Input: part model. Units: mm. Frame: model coordinates. Face numbers are marked on the shaded views. A direction names the side the tool comes from. Give positions to 0.01 mm unless a question says otherwise; leave off trailing zeros. Order: outer loops, then holes, each group sorted by start corner. A loop starts at its lowest first (then second) coordinate and runs counter-clockwise, first axis right, second up. Notation, with made-up numbers: (-21.5, -36) - (10.5, -36) arc R19 cw to (10.5, -23) - close; hole circle Ø6 at (-34, 2). An arc over 180 degrees is marked (long way). Answer in a Markdown table with one row per item. Add a question column.
1. Mould query, pull axis X, two halves, no side actions, for the marked faces 1 and 2. Classes: released by +X, released by -X, zero draft, split by the parting line, or undercut.
2. Access query for the marked faces 3, 4 and 5. Directions: +Z, -Z, +X, -X, +Y, -Y. A direction counts if a zero-diameter tool reaches every point of the face in a straight line with its end or side. Return the directions, or none.
3. Ray query, line 1 (X direction, y = 2.5, z = 0); line 2 (Y direction, x = -11.5, z = -3.5); line 3 (X direction, y = -2.5, z = 0). Return the intervals inside material, ascending. Write a range as [from, to].
4. Section query B-B on z = 0. Return loops of the section in (x, y), and give its area (3 significant figures).
5. Section query C-C on y = -3.75. Return loops of the section in (x, z).
6. Section query A-A on x = 0. Return loops of the section in (y, z), and give its area (3 significant figures).
7. Contact query for flat-ended pins moving along their axis: pin 1 (2 mm diameter, centred on x = 3, y = 2.5, fed in from -Z); pin 2 (2 mm diameter, centred on x = -0.5, y = 3.5, fed in from -Z); pin 3 (6 mm diameter, centred on y = 8, z = 9, fed in from -X). Output: stop coordinate, or through.
8. Section query D-D on z = 10.5. Return loops of the section in (x, y).
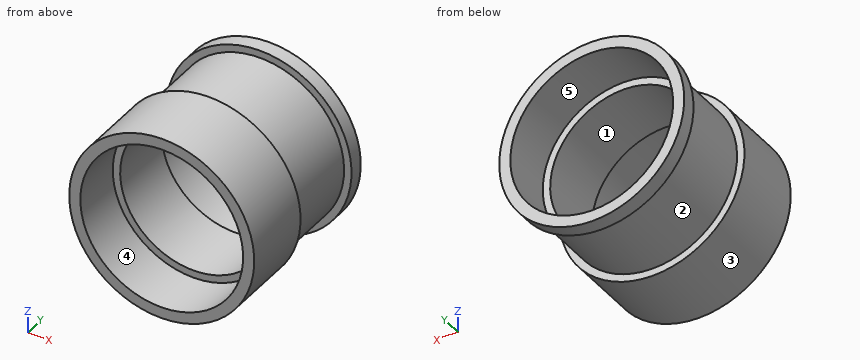
```python
from build123d import *

# Parameters (mm, degrees)
CROQUIS1_R                 = 12.5
SALIENTE_EXTRUIR1_DEPTH    = 11.5
CROQUIS2_R                 = 11
CORTAR_EXTRUIR1_DEPTH      = 7
CORTAR_EXTRUIR2_DEPTH      = 22.089096709
CORTAR_EXTRUIR2_DEPTH_BACK = 22.089096709
CROQUIS3_R                 = 10
CROQUIS4_W                 = 1
CROQUIS4_H                 = 11


with BuildPart() as part:
    # Croquis1 → Saliente-Extruir1 (new, symmetric)
    with BuildSketch(Plane(origin=(0, 0, 0), x_dir=(1, 0, 0), z_dir=(0, 1, 0))):
        with Locations(Location((0, 0, 0), (0, 0, 270))):
            Circle(CROQUIS1_R)
    extrude(amount=SALIENTE_EXTRUIR1_DEPTH, both=True)

    # Croquis2 → Cortar-Extruir1 (cut)
    with BuildSketch(Plane(origin=(0, 11.5, 0), x_dir=(1, 0, 0), z_dir=(0, 1, 0))):
        with Locations(Location((0, 0, 0), (0, 0, 270))):
            Circle(CROQUIS2_R)
    cortar_extruir1 = extrude(amount=-CORTAR_EXTRUIR1_DEPTH, mode=Mode.SUBTRACT)

    # Croquis3 → Cortar-Extruir2 (cut, two sides: drawn at the far end of the back side and taken through both)
    with BuildSketch(Plane(origin=(0, 0, 0), x_dir=(1, 0, 0), z_dir=(0, 1, 0)).offset(-CORTAR_EXTRUIR2_DEPTH_BACK)):
        with Locations(Location((0, 0, 0), (0, 0, 270))):
            Circle(CROQUIS3_R)
    extrude(amount=CORTAR_EXTRUIR2_DEPTH + CORTAR_EXTRUIR2_DEPTH_BACK, mode=Mode.SUBTRACT)

    # Simetría1: Cortar-Extruir1 across plane
    add(cortar_extruir1.mirror(Plane.ZX), mode=Mode.SUBTRACT)

    # Croquis4 → Cortar-Revolución1 (revolve, cut)
    with BuildSketch(Plane.XY, mode=Mode.PRIVATE) as cortar_revoluci_n1_sk:
        with Locations((12, 4)):
            Rectangle(CROQUIS4_W, CROQUIS4_H)
    revolve(cortar_revoluci_n1_sk.sketch.rotate(Axis((0, -12.65, 0), (0, 1, 0)), 90), axis=Axis((0, -12.65, 0), (0, 1, 0)), mode=Mode.SUBTRACT)


solid = part.part
```
Answer:
| question | item | result |
|---|---|---|
| 1 | face 1 | undercut |
| 1 | face 2 | split by the parting line |
| 2 | face 3 | +Y, -Y |
| 2 | face 4 | -Y |
| 2 | face 5 | +Y |
| 3 | line 1 | x = [-11.5, -10], [10, 11.5] |
| 3 | line 2 | y = [-11.5, -1.5], [9.5, 11.5] |
| 3 | line 3 | x = [-12.5, -10], [10, 12.5] |
| 4 | outline | (-12.5, -11.5) - (-11, -11.5) - (-11, -4.5) - (-10, -4.5) - (-10, 4.5) - (-11, 4.5) - (-11, 11.5) - (-12.5, 11.5) - (-12.5, 9.5) - (-11.5, 9.5) - (-11.5, -1.5) - (-12.5, -1.5) - close; (10, -4.5) - (11, -4.5) - (11, -11.5) - (12.5, -11.5) - (12.5, -1.5) - (11.5, -1.5) - (11.5, 9.5) - (12.5, 9.5) - (12.5, 11.5) - (11, 11.5) - (11, 4.5) - (10, 4.5) - close |
| 4 | area | 65.0 mm² |
| 5 | outline | circle Ø25 at (0, 0); hole circle Ø20 at (0, 0) |
| 6 | outline | (-11.5, -12.5) - (-1.5, -12.5) - (-1.5, -11.5) - (9.5, -11.5) - (9.5, -12.5) - (11.5, -12.5) - (11.5, -11) - (4.5, -11) - (4.5, -10) - (-4.5, -10) - (-4.5, -11) - (-11.5, -11) - close; (-11.5, 11) - (-4.5, 11) - (-4.5, 10) - (4.5, 10) - (4.5, 11) - (11.5, 11) - (11.5, 12.5) - (9.5, 12.5) - (9.5, 11.5) - (-1.5, 11.5) - (-1.5, 12.5) - (-11.5, 12.5) - close |
| 6 | area | 65.0 mm² |
| 7 | pin 1 | stops at z = -11.32 |
| 7 | pin 2 | stops at z = -11.5 |
| 7 | pin 3 | stops at x = -10.74 |
| 8 | outline | (-6.78, -11.5) - (-3.28, -11.5) - (-3.28, -4.5) - (3.28, -4.5) - (3.28, -11.5) - (6.78, -11.5) - (6.78, -1.5) - (4.69, -1.5) - (4.69, 9.5) - (6.78, 9.5) - (6.78, 11.5) - (3.28, 11.5) - (3.28, 4.5) - (-3.28, 4.5) - (-3.28, 11.5) - (-6.78, 11.5) - (-6.78, 9.5) - (-4.69, 9.5) - (-4.69, -1.5) - (-6.78, -1.5) - close |
